Could you check a few things on this model? Use its own coordinates, in mm. Coordinates: 2 decimals unless noted, no trailing zeros. Loops run counter-clockwise (first coordinate to the right, second up) from the corner with the lowest first, then second, coordinate; pieces in that order, holes last.
1) Imagine slicing it at B-B on y = 0.5. Please give me the cut outline in (x, z), plus the area to 3 significant figures.
2) Imagine slicing it at A-A on z = 5. Please give me the cut outline in (x, y), plus the area to 3 significant figures.
3) Will this pin go through, and if not, where does the flat tip stop? P1, Ø4, axis at x = 0, z = 5, coming from the -Y side.
4) If I drill on line 1 along Z through (x, y) = (0, -4.3); line 2 along Y through (x, z) = (3.25, 36); line 3 along X through (y, z) = (4.3, 5), over which ranges is the centre line in solid material (lowest first)?
5) Imagine slicing it at C-C on z = 45. Please give me the cut outline in (x, y).
6) Imagine slicing it at D-D on x = -0.75. Please give me the cut outline in (y, z), plus the area to 3 significant figures.
```python
from build123d import *

# Parameters (mm, degrees)
SKETCH_1_W          = 9
SKETCH_1_H          = 9
EXTRUDE_1_DEPTH     = 63
SKETCH_2_W          = 7
SKETCH_2_H          = 7
CUT_EXTRUDE_1_DEPTH = 83
SKETCH_3_R          = 2.2
SKETCH_3_R_2        = 1.5
CUT_EXTRUDE_2_DEPTH = 93


with BuildPart() as part:
    # ｽｹｯﾁ1 → ﾎﾞｽ - 押し出し1 (new body)
    with BuildSketch(Plane.XY):
        Rectangle(SKETCH_1_W, SKETCH_1_H)
    extrude(amount=EXTRUDE_1_DEPTH)

    # ｽｹｯﾁ2 → ｶｯﾄ - 押し出し1 (cut)
    with BuildSketch(Plane.XY.offset(63)):
        Rectangle(SKETCH_2_W, SKETCH_2_H)
    extrude(amount=-CUT_EXTRUDE_1_DEPTH, mode=Mode.SUBTRACT)

    # ｽｹｯﾁ3 → ｶｯﾄ - 押し出し2 (cut)
    with BuildSketch(Plane(origin=(0, 4.5, 0), x_dir=(1, 0, 0), z_dir=(0, 1, 0))):
        with Locations((0, -5)):
            Circle(SKETCH_3_R)
        with Locations((0, -58)):
            Circle(SKETCH_3_R_2)
    extrude(amount=-CUT_EXTRUDE_2_DEPTH, mode=Mode.SUBTRACT)


solid = part.part
```
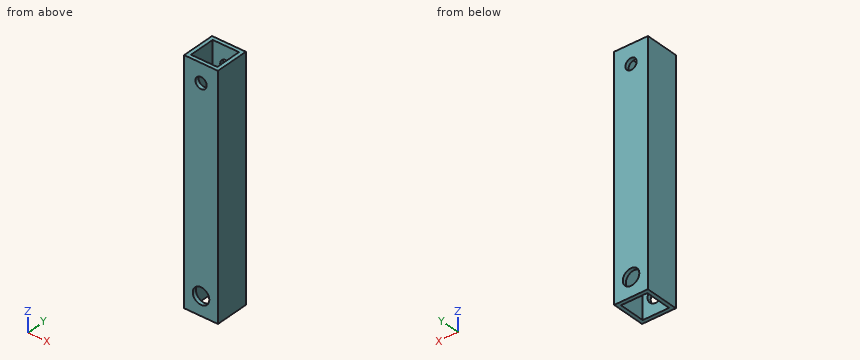
Filled in:
1. outline: (-4.5, 0) - (-3.5, 0) - (-3.5, 63) - (-4.5, 63) - close; (3.5, 0) - (4.5, 0) - (4.5, 63) - (3.5, 63) - close
1. area: 126 mm2
2. outline: (-4.5, -4.5) - (-2.2, -4.5) - (-2.2, -3.5) - (-3.5, -3.5) - (-3.5, 3.5) - (-2.2, 3.5) - (-2.2, 4.5) - (-4.5, 4.5) - close; (2.2, -4.5) - (4.5, -4.5) - (4.5, 4.5) - (2.2, 4.5) - (2.2, 3.5) - (3.5, 3.5) - (3.5, -3.5) - (2.2, -3.5) - close
2. area: 23.2 mm2
3. P1: passes through
4. line 1: z = 0 to 2.8, 7.2 to 56.5, 59.5 to 63
4. line 2: y = -4.5 to -3.5, 3.5 to 4.5
4. line 3: x = -4.5 to -2.2, 2.2 to 4.5
5. outline: (-4.5, -4.5) - (4.5, -4.5) - (4.5, 4.5) - (-4.5, 4.5) - close; hole (-3.5, -3.5) - (3.5, -3.5) - (3.5, 3.5) - (-3.5, 3.5) - close
6. outline: (-4.5, 0) - (-3.5, 0) - (-3.5, 2.93) - (-4.5, 2.93) - close; (-4.5, 7.07) - (-3.5, 7.07) - (-3.5, 56.7) - (-4.5, 56.7) - close; (-4.5, 59.3) - (-3.5, 59.3) - (-3.5, 63) - (-4.5, 63) - close; (3.5, 0) - (4.5, 0) - (4.5, 2.93) - (3.5, 2.93) - close; (3.5, 7.07) - (4.5, 7.07) - (4.5, 56.7) - (3.5, 56.7) - close; (3.5, 59.3) - (4.5, 59.3) - (4.5, 63) - (3.5, 63) - close
6. area: 113 mm2
